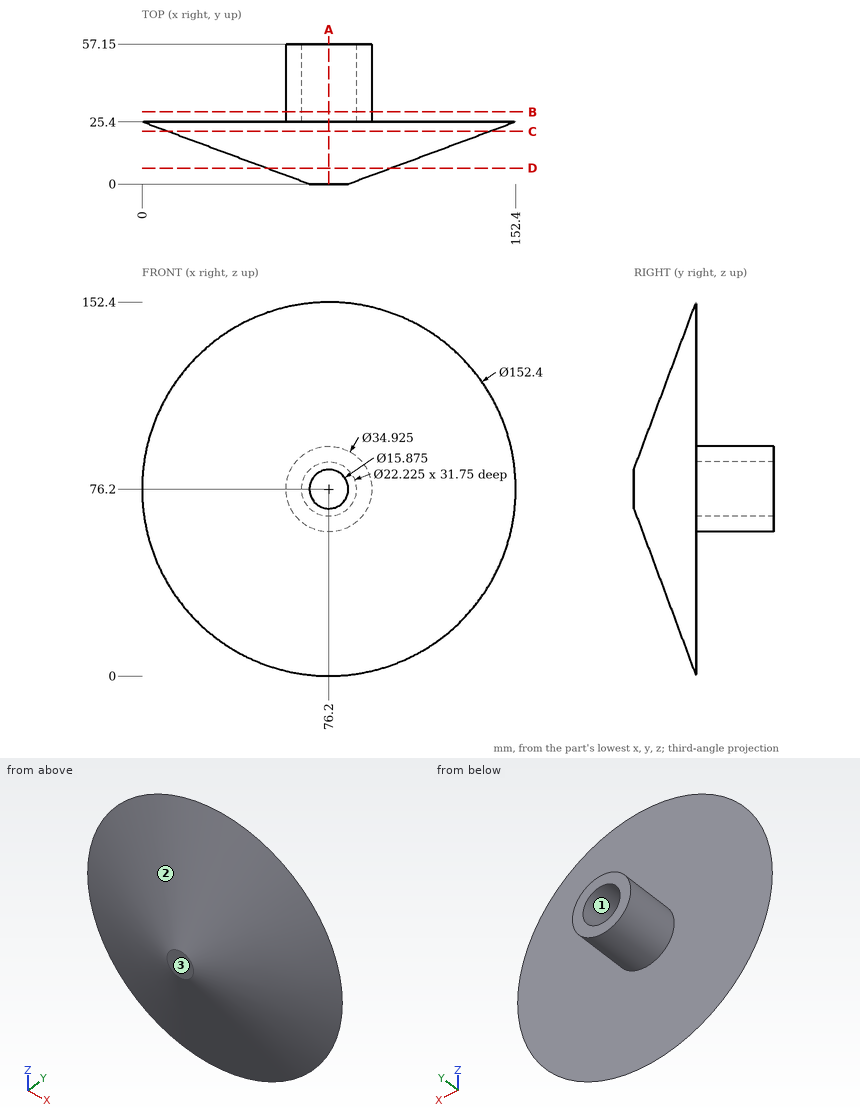
The figure shows three views and two pictorial views of one solid part (mm, origin at its lowest corner). Answer the questions. Give positions to 0.01 mm unless a question says otherwise; leave off trailing zeros. Order: outer loops, then holes, each group sorted by start corner. A loop starts at its lowest first (then second) coordinate and runs counter-clockwise, first axis right, second up. Notation, with made-up numbers: M -5.5,66 L 10.5,66 A10 ccw 10.5,77 Z; hole C -22,64 d4. An arc over 180 degrees is marked long. Return JSON: item names as keys, results as strings.
1) Section D-D, the plane y = 6.5 is taken. Write down the section's boundary in (x, z), plus the area to 3 significant figures.
Resolved:
{"outline": "C 76.2,76.2 d50.81", "area": "2,030 mm^2"}
2) Section C-C, the plane y = 21.5 is taken. Write down the section's boundary in (x, z), plus the area to 3 significant figures.
Resolved:
{"outline": "C 76.2,76.2 d131.44", "area": "13,600 mm^2"}
3) For a pull along Z with two mould halves and no side action, classify the marked faces 1, 2 and 3 as +Z half, -Z half, draft (parallel to the pull), parting line (faces both ways), or undercut.
Resolved:
{"face 1": "undercut", "face 2": "parting line", "face 3": "draft"}
4) Straight lines are drawn through the part: line 1 along Z through (x, y) = (76.2, 42); line 2 along Y through (x, z) = (83, 74); line 3 along X through (y, z) = (41.5, 75). For each, find the intervals that lie inside material, in ascending order. Write a range as [from, to].
Resolved:
{"line 1": "[58.74, 65.09], [87.31, 93.66]", "line 2": "[0, 25.4]", "line 3": "[58.78, 65.15], [87.25, 93.62]"}
5) Section B-B, the plane y = 29.5 is taken. Write down the section's boundary in (x, z) (1 decimal).
Resolved:
{"outline": "C 76.2,76.2 d34.9; hole C 76.2,76.2 d22.2"}
6) Each of these flat-tipped pins is pushed along its axis until it touches: pin 1 (1.5 mm diameter, centred on y = 27.5, z = 71.5, fed in from +X); pin 2 (1.5 mm diameter, centred on x = 85.5, z = 53.5, fed in from -Y); pin 3 (11 mm diameter, centred on x = 78, z = 77.5, fed in from +Y). Where does it stop, or does it pass through?
Resolved:
{"pin 1": "x = 93.21", "pin 2": "y = 5.9", "pin 3": "y = 25.4"}
7) Section A-A, the plane x = 76.2 is taken. Write down the section's boundary in (y, z).
Resolved:
{"outline": "M 0,68.26 L 25.4,0 L 25.4,58.74 L 57.15,58.74 L 57.15,65.09 L 25.4,65.09 L 25.4,87.31 L 57.15,87.31 L 57.15,93.66 L 25.4,93.66 L 25.4,152.4 L 0,84.14 Z"}
